```python
from build123d import *

# Parameters (mm, degrees)
SKETCH_1_R               = 10.25
EXTRUDE_1_DEPTH          = 20
SKETCH_2_R               = 4.5
CUT_EXTRUDE_1_DEPTH      = 20
CUT_EXTRUDE_2_DEPTH      = 1
CUT_EXTRUDE_2_DEPTH_BACK = 37
CHAMFER_1_SIZE           = 1


with BuildPart() as part:
    # 草图1 → 凸台-拉伸1 (new body, symmetric)
    with BuildSketch(Plane.XY):
        with BuildLine():
            Line((0, -80), (18, -80))
            Line((18, -80), (18, -15))
            Line((18, -15), (15, 0))
            ThreePointArc((15, 0), (0, 15), (-15, 0))
            Line((-15, 0), (-18, -15))
            Line((-18, -15), (-18, -80))
            Line((-18, -80), (0, -80))
        make_face()
        Circle(SKETCH_1_R, mode=Mode.SUBTRACT)
    extrude(amount=EXTRUDE_1_DEPTH, both=True)

    # 草图2 → 切除-拉伸1 (cut, symmetric)
    with BuildSketch(Plane(origin=(0, 0, 0), x_dir=(0, 0, -1), z_dir=(1, 0, 0))):
        with Locations((0, -45)):
            Circle(SKETCH_2_R)
        with Locations((0, -25)):
            Circle(SKETCH_2_R)
        with Locations((0, -65)):
            Circle(SKETCH_2_R)
    extrude(amount=CUT_EXTRUDE_1_DEPTH, both=True, mode=Mode.SUBTRACT)

    # 草图7 → 切除-拉伸2 (cut, two sides)
    with BuildSketch(Plane(origin=(18, 0, 0), x_dir=(0, 0, -1), z_dir=(1, 0, 0))) as cut_extrude_2_sk:
        with BuildLine():
            Line((-15, -65), (-20, -45))
            Line((-20, -45), (-20, -80))
            Line((-20, -80), (1.38e-07, -80))
            ThreePointArc((1.38e-07, -80), (-10.606601669, -75.606601767), (-15, -65))
        make_face()
        with BuildLine():
            ThreePointArc((15, -65), (10.606601767, -75.606601669), (1.38e-07, -80))
            Line((1.38e-07, -80), (20, -80))
            Line((20, -80), (20, -45))
            Line((20, -45), (15, -65))
        make_face()
    extrude(amount=CUT_EXTRUDE_2_DEPTH, mode=Mode.SUBTRACT)
    extrude(cut_extrude_2_sk.sketch, amount=-CUT_EXTRUDE_2_DEPTH_BACK, mode=Mode.SUBTRACT)

    # 倒角1
    chamfer_1_edges = [part.edges().sort_by_distance(p)[0] for p in [
        (16.5, -7.5, 20),
        (-10.25, 0, -20),
        (-10.25, 0, 20),
        (0, 15, 20),
        (-16.5, -7.5, 20),
        (-18, -30, 20),
        (-18, -55, -17.5),
        (-18, -80, 0),
        (-18, -55, 17.5),
        (18, -30, -20),
        (18, -30, 20),
        (18, -55, 17.5),
        (18, -80, 0),
        (18, -55, -17.5),
        (-18, -30, -20),
        (-16.5, -7.5, -20),
        (0, 15, -20),
        (16.5, -7.5, -20),
    ]]
    chamfer(chamfer_1_edges, length=CHAMFER_1_SIZE)


solid = part.part
```
Here's how the part is built. I have some questions about the finished solid (model axes, mm). Round coordinates to 2 decimals unless told otherwise and drop trailing zeros. Write each loop counter-clockwise with the first axis right and the second up, starting at its lowest first coordinate (ties: lowest second). Pieces come first, ordered by that corner, then holes.
Q1. Will these pins go through, and if not, where does the flat tip stop? P1, Ø1, axis at x = 8, z = -12.5, coming from the +Y side; P2, Ø2, axis at x = -4, y = -60.5, coming from the -Z side (3 decimals); P3, Ø8, axis at x = -6.5, z = 8.5, coming from the +Y side.
Q2. If we section it at A-A on y = -25: Write out the boundary of the cut face in (x, z).
Q3. If we section it at B-B on x = 2: Give the number of separate pieces and of enclosed holes in the cut face, plus the area to 3 significant figures.
Q4. Please list where these lines run through material, in increasing order: probe 1 along Z at (x, y) = (10, -45); probe 2 along Z at (x, y) = (-13, -47); probe 3 along Y at (x, z) = (2, -5.5).
Q5. If we mould it in two halves opening along Y, with no side actions, what happens to faces 1 (the cylindrical face through (0.25, -60.54, 0.59)), 2 (the cylindrical face through (0, 15, 0)), 3 (the flat face through (-17.507, -55.079, -16.958))? For each: +Y half, -Y half, draft (parallel to the pull), parting line (faces both ways), or undercut.
Answer below:
1. P1: stops at y = 12.99
1. P2: stops at z = -16.375
1. P3: stops at y = 14.79
2. outline: (-18, -19) - (-17, -20) - (17, -20) - (18, -19) - (18, -4.5) - (-18, -4.5) - close; (-18, 4.5) - (18, 4.5) - (18, 19) - (17, 20) - (-17, 20) - (-18, 19) - close
3. separate pieces: 2
3. enclosed holes: 3
3. area: 2,450 mm2
4. probe 1: z = -20 to -4.5, 4.5 to 20
4. probe 2: z = -19.5 to -4.03, 4.03 to 19.5
4. probe 3: y = -78.96 to -10.05, 10.05 to 14.87
5. face 1: undercut
5. face 2: +Y half
5. face 3: -Y half
